from build123d import *

# Parameters (mm, degrees)
SKETCH1_R               = 32.5
SKETCH1_W               = 120.65
SKETCH1_H               = 50.8
BOSS_EXTRUDE2_DEPTH     = 6.35
BOSS_EXTRUDE3_START     = 6.35
SKETCH1_3_R             = 32.5
BOSS_EXTRUDE3_DEPTH     = 25.4
CUT_EXTRUDE1_DEPTH      = 170.176810751
CUT_EXTRUDE1_DEPTH_BACK = 170.176810751
SKETCH2_R               = 3.175
SKETCH3_R               = 6.35
CUT_EXTRUDE2_DEPTH      = 25.4
SKETCH4_3_R             = 4.7625
CUT_EXTRUDE3_DEPTH      = 6.35
FILLET1_R               = 12.7
SKETCH5_R               = 32.5
SKETCH5_R_2             = 30.849
BOSS_EXTRUDE6_DEPTH     = 1.5875


with BuildPart() as part:
    # Sketch1 → Boss-Extrude2 (new body)
    # profile 1 of 2: a face of its own
    with BuildSketch(Plane.XY):
        with BuildLine():
            Line((32.171066193, 31.75), (161.036, 31.75))
            Line((161.036, 31.75), (161.036, 25.4))
            Line((161.036, 25.4), (40.386, 25.4))
            Line((40.386, 25.4), (40.386, -25.4))
            Line((40.386, -25.4), (161.036, -25.4))
            Line((161.036, -25.4), (161.036, -31.75))
            Line((161.036, -31.75), (32.171066193, -31.75))
            ThreePointArc((32.171066193, -31.75), (-45.2, 0), (32.171066193, 31.75))
        make_face()
        Circle(SKETCH1_R, mode=Mode.SUBTRACT)
    # profile 2 of 2: a face of its own
    with BuildSketch(Plane.XY):
        with Locations((100.711, 0)):
            Rectangle(SKETCH1_W, SKETCH1_H)
    extrude(amount=BOSS_EXTRUDE2_DEPTH)

    # Sketch1<3> → Boss-Extrude3 (add)
    with BuildSketch(Plane.XY.offset(BOSS_EXTRUDE3_START)):
        with BuildLine():
            Line((32.171066193, 31.75), (161.036, 31.75))
            Line((161.036, 31.75), (161.036, 25.4))
            Line((161.036, 25.4), (40.386, 25.4))
            Line((40.386, 25.4), (40.386, -25.4))
            Line((40.386, -25.4), (161.036, -25.4))
            Line((161.036, -25.4), (161.036, -31.75))
            Line((161.036, -31.75), (32.171066193, -31.75))
            ThreePointArc((32.171066193, -31.75), (-45.2, 0), (32.171066193, 31.75))
        make_face()
        Circle(SKETCH1_3_R, mode=Mode.SUBTRACT)
    extrude(amount=BOSS_EXTRUDE3_DEPTH)

    # Sketch2 → Cut-Extrude1 (cut, two sides: drawn at the far end of the back side and taken through both)
    with BuildSketch(Plane.XY.offset(6.35).offset(-CUT_EXTRUDE1_DEPTH_BACK)):
        with Locations((49.911, 15.875)):
            Circle(SKETCH2_R)
        with Locations((151.511, 15.875)):
            Circle(SKETCH2_R)
        with Locations((151.511, -15.875)):
            Circle(SKETCH2_R)
        with Locations((49.911, -15.875)):
            Circle(SKETCH2_R)
        with Locations((27.471098449, 27.471098449)):
            Circle(SKETCH2_R)
        with Locations((27.471098449, -27.471098449)):
            Circle(SKETCH2_R)
        with Locations((-27.471098449, -27.471098449)):
            Circle(SKETCH2_R)
        with Locations((-27.471098449, 27.471098449)):
            Circle(SKETCH2_R)
    extrude(amount=CUT_EXTRUDE1_DEPTH + CUT_EXTRUDE1_DEPTH_BACK, mode=Mode.SUBTRACT)

    # Sketch3 → Cut-Extrude2 (cut)
    with BuildSketch(Plane.XY.offset(31.75)):
        with Locations((44.876128061, 20.909871939)):
            Circle(SKETCH3_R)
        with Locations((44.876128061, -20.909871939)):
            Circle(SKETCH3_R)
    extrude(amount=-CUT_EXTRUDE2_DEPTH, mode=Mode.SUBTRACT)

    # Sketch4<3> → Cut-Extrude3 (cut)
    with BuildSketch(Plane(origin=(0, 0, 0), x_dir=(-1, 0, 0), z_dir=(0, 0, -1))):
        with Locations((-63.5, 0)):
            Circle(SKETCH4_3_R)
    extrude(amount=-CUT_EXTRUDE3_DEPTH, mode=Mode.SUBTRACT)

    # Fillet1
    fillet1_edges = [part.edges().sort_by_distance(p)[0] for p in [
        (32.171066193, -31.75, 15.875),
        (32.171066193, 31.75, 15.875),
    ]]
    fillet(fillet1_edges, radius=FILLET1_R)

    # Sketch5 → Boss-Extrude6 (add)
    with BuildSketch(Plane(origin=(0, 0, 0), x_dir=(-1, 0, 0), z_dir=(0, 0, -1))):
        Circle(SKETCH5_R)
        Circle(SKETCH5_R_2, mode=Mode.SUBTRACT)
    extrude(amount=-BOSS_EXTRUDE6_DEPTH)


solid = part.part
For this review, take the finished solid that the model builds, in its own axes (mm). A direction names the side the tool comes from. Round coordinates to 2 decimals unless told otherwise and drop trailing zeros. Loops run counter-clockwise (first coordinate to the right, second up) from the corner with the lowest first, then second, coordinate; pieces in that order, holes last. Notation, with made-up numbers: (52.5, -31.5) - (97.5, -31.5) arc R10 ccw to (97.5, -26.5) - close; hole circle Ø11 at (73, -36). An arc over 180 degrees is marked (long way). One line per item, written item: value. Start each with the question number.
Item 1: For faces 1 (the flat face through (100, -31.75, 16)), 2 (the flat face through (104, -25.4, 19)), 3 (the cylindrical face through (31, 9.76, 16.46)), list the 3-axis set-ups (+Z, -Z, +X, -X, +Y, -Y) from which the entire face can be reached by the end or side of a thin tool; tool diameter is ignored.
Item 2: Clearance check with flat-ended pins moving along their axes: pin 1 Ø5 at (x, z) = (91.5, 6) entering from -Y; pin 2 Ø4 at (y, z) = (-13, 5) entering from -X; pin 3 Ø3 at (x, y) = (121, 23.5) entering from +Z; pin 4 Ø4 at (x, y) = (49.911, 15.875) entering from -Z. State where each tip first meets the part, or that it passes through.
Item 3: Take a section at B-B (y = 0). Give the boundary of the cut face in (x, z), plus the area to 3 significant figures.
Item 4: Take a section at A-A (x = 0). Give the boundary of the cut face in (y, z).
Item 5: Take a section at C-C (x = 90.5). Give the boundary of the cut face in (y, z).
Item 6: Take a section at D-D (y = -22). Give the boundary of the cut face in (x, z), plus the area to 3 significant figures.
Item 7: For L1, parallel to X at y = -0.5, z = 6; L2, parallel to Y at x = 0, z = 1.2; L3, parallel to Y at x = 78, z = 24, list the stretches that pass through material, from the lowest coordinate up.
Item 8: The part is to be moulded in two halves that separate along X. For faces 4 (the flat face through (40.386, 0, 19)), 5 (the cylindrical face through (40.49, 25.5, 19.23)), 6 (the cylindrical face through (-45.177, -1.434, 15.653)), say which applies: +X half, -X half, draft (parallel to the pull), parting line (faces both ways), or undercut.
Answer below:
1. face 1: +Z, -Z, +X, -Y
1. face 2: +Z, +X
1. face 3: +Z
2. pin 1: stops at y = -31.75
2. pin 2: stops at x = -43.84
2. pin 3: stops at z = 6.35
2. pin 4: passes through
3. outline: (-45.2, 0) - (-30.85, 0) - (-30.85, 1.59) - (-32.5, 1.59) - (-32.5, 31.75) - (-45.2, 31.75) - close; (30.85, 0) - (58.74, 0) - (58.74, 6.35) - (40.39, 6.35) - (40.39, 31.75) - (32.5, 31.75) - (32.5, 1.59) - (30.85, 1.59) - close; (68.26, 0) - (161.04, 0) - (161.04, 6.35) - (68.26, 6.35) - close
3. area: 1,360 mm2
4. outline: (-45.2, 0) - (-30.85, 0) - (-30.85, 1.59) - (-32.5, 1.59) - (-32.5, 31.75) - (-45.2, 31.75) - close; (30.85, 0) - (45.2, 0) - (45.2, 31.75) - (32.5, 31.75) - (32.5, 1.59) - (30.85, 1.59) - close
5. outline: (-31.75, 0) - (31.75, 0) - (31.75, 31.75) - (25.4, 31.75) - (25.4, 6.35) - (-25.4, 6.35) - (-25.4, 31.75) - (-31.75, 31.75) - close
6. outline: (-39.48, 0) - (-21.63, 0) - (-21.63, 1.59) - (-23.92, 1.59) - (-23.92, 31.75) - (-39.48, 31.75) - close; (21.63, 0) - (161.04, 0) - (161.04, 6.35) - (38.62, 6.35) - (38.62, 31.75) - (23.92, 31.75) - (23.92, 1.59) - (21.63, 1.59) - close
6. area: 1,750 mm2
7. L1: x = -45.2 to -32.5, 32.5 to 58.76, 68.24 to 161.04
7. L2: y = -45.2 to -30.85, 30.85 to 45.2
7. L3: y = -31.75 to -25.4, 25.4 to 31.75
8. face 4: +X half
8. face 5: undercut
8. face 6: parting line
